from build123d import *

# Parameters (mm, degrees)
F0_W         = 61.9125
F0_H         = 25.4
F1_DEPTH     = 73.025
F3_T         = -2.54
F4_W         = 56.8325
F4_H         = 67.945
F5_DEPTH     = 2.54
F6_T1_DEPTH  = 50.8
F6_T3_DEPTH  = 87.3125
F6_T8_DEPTH  = 87.3125
F6_T14_DEPTH = 87.3125
F6_T20_DEPTH = 87.3125
F6_T27_DEPTH = 87.3125
F6_T33_DEPTH = 87.3125
F7_T1_DEPTH  = 50.8
F7_T3_DEPTH  = 87.3125
F7_T8_DEPTH  = 87.3125
F7_T14_DEPTH = 87.3125
F7_T20_DEPTH = 87.3125
F7_T27_DEPTH = 87.3125
F7_T33_DEPTH = 87.3125
F2_R         = 4.7625
F8_DEPTH     = 61.9135
F10_DEPTH    = 19.05


# Not quite as in the source:
# - a fillet or chamfer that OpenCascade refuses, or shapes differently, is made with other operations: its cross-section is extruded or revolved along the edge and cut away or added


with BuildPart() as f1:
    # F0 (on Front) → F1 (new body)
    with BuildSketch(Plane.XZ):
        Rectangle(F0_W, F0_H)
    extrude(amount=F1_DEPTH)

    # F3
    f3_openings = [f1.faces().sort_by_distance(p)[0] for p in [
        (0, -36.5125, -12.7),
    ]]
    offset(amount=F3_T, openings=f3_openings)

    # F4 (on face) → F5 (join)
    with BuildSketch(Plane.XY.offset(12.7)):
        with Locations((0, -36.5125)):
            Rectangle(F4_W, F4_H)
    extrude(amount=F5_DEPTH)

    # F6: fillet of radius 5.08 on 4 edges, made by hand

    # F6_s2 → F6_t1 (cut)
    with BuildSketch(Plane.XY.offset(-25.4)):
        with BuildLine():
            ThreePointArc((-25.87625, 0), (-29.4683524484, -1.4878975516), (-30.95625, -5.08))
            Line((-30.95625, -5.08), (-30.95625, 0))
            Line((-30.95625, 0), (-25.87625, 0))
        make_face()
        with BuildLine():
            ThreePointArc((30.95625, -5.08), (29.4683524484, -1.4878975516), (25.87625, 0))
            Line((25.87625, 0), (30.95625, 0))
            Line((30.95625, 0), (30.95625, -5.08))
        make_face()
    extrude(amount=F6_T1_DEPTH, mode=Mode.SUBTRACT)

    # F6_s4 → F6_t3 (cut)
    with BuildSketch(Plane.YZ.offset(-43.65625)):
        with BuildLine():
            ThreePointArc((0, -7.62), (-1.4878975516, -11.2121024484), (-5.08, -12.7))
            Line((-5.08, -12.7), (0, -12.7))
            Line((0, -12.7), (0, -7.62))
        make_face()
    extrude(amount=F6_T3_DEPTH, mode=Mode.SUBTRACT)


with BuildPart() as f6_tool6:
    # F6_s7 → F6_t8 (new body)
    with BuildSketch(Plane.YZ.offset(43.65625)):
        with BuildLine():
            ThreePointArc((-5.08, 12.7), (-1.4878975516, 11.2121024484), (0, 7.62))
            Line((0, 7.62), (0, 12.7))
            Line((0, 12.7), (-5.08, 12.7))
        make_face()
    extrude(amount=-F6_T8_DEPTH)

    split(bisect_by=Plane.XZ.offset(2.54), keep=Keep.TOP)

    split(bisect_by=Plane.YZ.offset(28.41625), keep=Keep.TOP)


with BuildPart() as f1_1:
    add(f1.part)

    # F6_t5: cut F6_tool6
    add(f6_tool6.part, mode=Mode.SUBTRACT)


with BuildPart() as f6_tool12:
    # F6_s13 → F6_t14 (new body)
    with BuildSketch(Plane.YZ.offset(43.65625)):
        with BuildLine():
            ThreePointArc((-5.08, 12.7), (-1.4878975516, 11.2121024484), (0, 7.62))
            Line((0, 7.62), (0, 12.7))
            Line((0, 12.7), (-5.08, 12.7))
        make_face()
    extrude(amount=-F6_T14_DEPTH)

    split(bisect_by=Plane.XZ.offset(2.54), keep=Keep.BOTTOM)

    split(bisect_by=Plane.YZ.offset(28.41625), keep=Keep.TOP)


with BuildPart() as f1_2:
    add(f1_1.part)

    # F6_t11: cut F6_tool12
    add(f6_tool12.part, mode=Mode.SUBTRACT)


with BuildPart() as f6_tool18:
    # F6_s19 → F6_t20 (new body)
    with BuildSketch(Plane.YZ.offset(43.65625)):
        with BuildLine():
            ThreePointArc((-5.08, 12.7), (-1.4878975516, 11.2121024484), (0, 7.62))
            Line((0, 7.62), (0, 12.7))
            Line((0, 12.7), (-5.08, 12.7))
        make_face()
    extrude(amount=-F6_T20_DEPTH)

    split(bisect_by=Plane.YZ.offset(-28.41625), keep=Keep.TOP)

    split(bisect_by=Plane.XZ.offset(2.54), keep=Keep.BOTTOM)

    split(bisect_by=Plane.YZ.offset(28.41625), keep=Keep.BOTTOM)


with BuildPart() as f1_3:
    add(f1_2.part)

    # F6_t17: cut F6_tool18
    add(f6_tool18.part, mode=Mode.SUBTRACT)


with BuildPart() as f6_tool25:
    # F6_s26 → F6_t27 (new body)
    with BuildSketch(Plane.YZ.offset(43.65625)):
        with BuildLine():
            ThreePointArc((-5.08, 12.7), (-1.4878975516, 11.2121024484), (0, 7.62))
            Line((0, 7.62), (0, 12.7))
            Line((0, 12.7), (-5.08, 12.7))
        make_face()
    extrude(amount=-F6_T27_DEPTH)

    split(bisect_by=Plane.YZ.offset(-28.41625), keep=Keep.BOTTOM)

    split(bisect_by=Plane.XZ.offset(2.54), keep=Keep.TOP)


with BuildPart() as f1_4:
    add(f1_3.part)

    # F6_t24: cut F6_tool25
    add(f6_tool25.part, mode=Mode.SUBTRACT)


with BuildPart() as f6_tool31:
    # F6_s32 → F6_t33 (new body)
    with BuildSketch(Plane.YZ.offset(43.65625)):
        with BuildLine():
            ThreePointArc((-5.08, 12.7), (-1.4878975516, 11.2121024484), (0, 7.62))
            Line((0, 7.62), (0, 12.7))
            Line((0, 12.7), (-5.08, 12.7))
        make_face()
    extrude(amount=-F6_T33_DEPTH)

    split(bisect_by=Plane.YZ.offset(-28.41625), keep=Keep.BOTTOM)

    split(bisect_by=Plane.XZ.offset(2.54), keep=Keep.BOTTOM)


with BuildPart() as f1_5:
    add(f1_4.part)

    # F6_t30: cut F6_tool31
    add(f6_tool31.part, mode=Mode.SUBTRACT)

    # F7: fillet of radius 5.08 on 4 edges, made by hand

    # F7_s2 → F7_t1 (cut)
    with BuildSketch(Plane.XY.offset(-25.4)):
        with BuildLine():
            ThreePointArc((-25.87625, -73.025), (-29.4683524484, -71.5371024484), (-30.95625, -67.945))
            Line((-30.95625, -67.945), (-30.95625, -73.025))
            Line((-30.95625, -73.025), (-25.87625, -73.025))
        make_face()
        with BuildLine():
            ThreePointArc((30.95625, -67.945), (29.4683524484, -71.5371024484), (25.87625, -73.025))
            Line((25.87625, -73.025), (30.95625, -73.025))
            Line((30.95625, -73.025), (30.95625, -67.945))
        make_face()
    extrude(amount=F7_T1_DEPTH, mode=Mode.SUBTRACT)

    # F7_s4 → F7_t3 (cut)
    with BuildSketch(Plane.YZ.offset(-43.65625)):
        with BuildLine():
            ThreePointArc((-67.945, -12.7), (-71.5371024484, -11.2121024484), (-73.025, -7.62))
            Line((-73.025, -7.62), (-73.025, -12.7))
            Line((-73.025, -12.7), (-67.945, -12.7))
        make_face()
    extrude(amount=F7_T3_DEPTH, mode=Mode.SUBTRACT)


with BuildPart() as f7_tool6:
    # F7_s7 → F7_t8 (new body)
    with BuildSketch(Plane.YZ.offset(43.65625)):
        with BuildLine():
            ThreePointArc((-67.945, 12.7), (-71.5371024484, 11.2121024484), (-73.025, 7.62))
            Line((-73.025, 7.62), (-73.025, 12.7))
            Line((-73.025, 12.7), (-67.945, 12.7))
        make_face()
    extrude(amount=-F7_T8_DEPTH)

    split(bisect_by=Plane.YZ.offset(28.41625), keep=Keep.TOP)

    split(bisect_by=Plane.XZ.offset(70.485), keep=Keep.BOTTOM)


with BuildPart() as f1_6:
    add(f1_5.part)

    # F7_t5: cut F7_tool6
    add(f7_tool6.part, mode=Mode.SUBTRACT)


with BuildPart() as f7_tool12:
    # F7_s13 → F7_t14 (new body)
    with BuildSketch(Plane.YZ.offset(43.65625)):
        with BuildLine():
            ThreePointArc((-67.945, 12.7), (-71.5371024484, 11.2121024484), (-73.025, 7.62))
            Line((-73.025, 7.62), (-73.025, 12.7))
            Line((-73.025, 12.7), (-67.945, 12.7))
        make_face()
    extrude(amount=-F7_T14_DEPTH)

    split(bisect_by=Plane.YZ.offset(28.41625), keep=Keep.TOP)

    split(bisect_by=Plane.XZ.offset(70.485), keep=Keep.TOP)


with BuildPart() as f1_7:
    add(f1_6.part)

    # F7_t11: cut F7_tool12
    add(f7_tool12.part, mode=Mode.SUBTRACT)


with BuildPart() as f7_tool18:
    # F7_s19 → F7_t20 (new body)
    with BuildSketch(Plane.YZ.offset(43.65625)):
        with BuildLine():
            ThreePointArc((-67.945, 12.7), (-71.5371024484, 11.2121024484), (-73.025, 7.62))
            Line((-73.025, 7.62), (-73.025, 12.7))
            Line((-73.025, 12.7), (-67.945, 12.7))
        make_face()
    extrude(amount=-F7_T20_DEPTH)

    split(bisect_by=Plane.YZ.offset(28.41625), keep=Keep.BOTTOM)

    split(bisect_by=Plane.XZ.offset(70.485), keep=Keep.TOP)

    split(bisect_by=Plane.YZ.offset(-28.41625), keep=Keep.TOP)


with BuildPart() as f1_8:
    add(f1_7.part)

    # F7_t17: cut F7_tool18
    add(f7_tool18.part, mode=Mode.SUBTRACT)


with BuildPart() as f7_tool25:
    # F7_s26 → F7_t27 (new body)
    with BuildSketch(Plane.YZ.offset(43.65625)):
        with BuildLine():
            ThreePointArc((-67.945, 12.7), (-71.5371024484, 11.2121024484), (-73.025, 7.62))
            Line((-73.025, 7.62), (-73.025, 12.7))
            Line((-73.025, 12.7), (-67.945, 12.7))
        make_face()
    extrude(amount=-F7_T27_DEPTH)

    split(bisect_by=Plane.XZ.offset(70.485), keep=Keep.BOTTOM)

    split(bisect_by=Plane.YZ.offset(-28.41625), keep=Keep.BOTTOM)


with BuildPart() as f1_9:
    add(f1_8.part)

    # F7_t24: cut F7_tool25
    add(f7_tool25.part, mode=Mode.SUBTRACT)


with BuildPart() as f7_tool31:
    # F7_s32 → F7_t33 (new body)
    with BuildSketch(Plane.YZ.offset(43.65625)):
        with BuildLine():
            ThreePointArc((-67.945, 12.7), (-71.5371024484, 11.2121024484), (-73.025, 7.62))
            Line((-73.025, 7.62), (-73.025, 12.7))
            Line((-73.025, 12.7), (-67.945, 12.7))
        make_face()
    extrude(amount=-F7_T33_DEPTH)

    split(bisect_by=Plane.XZ.offset(70.485), keep=Keep.TOP)

    split(bisect_by=Plane.YZ.offset(-28.41625), keep=Keep.BOTTOM)


with BuildPart() as f1_10:
    add(f1_9.part)

    # F7_t30: cut F7_tool31
    add(f7_tool31.part, mode=Mode.SUBTRACT)

    # F2 (on face) → F8 (cut, through all)
    with BuildSketch(Plane.YZ.offset(30.95625)):
        with Locations((-36.5125, 0)):
            Circle(F2_R)
    extrude(amount=-F8_DEPTH, mode=Mode.SUBTRACT)

    # F9 (on face) → F10 (join)
    with BuildSketch(Plane(origin=(0, 0, 10.16), x_dir=(1, 0, 0), z_dir=(0, 0, -1))):
        Polygon((-3.175, 61.9125), (3.175, 61.9125), (3.175, 59.2770799994), (6.35, 59.3725), (6.35, 61.9125), (6.35, 70.485), (0, 70.485), (-6.35, 70.485), (-6.35, 61.9125), (-6.35, 59.3725), (-3.175, 59.3725), align=None)
        Polygon((3.175, 13.6525), (3.175, 11.1125), (-3.175, 11.1125), (-3.175, 13.6525), (-6.35, 13.6525), (-6.35, 11.1125), (-6.35, 2.54), (6.35, 2.54), (6.35, 11.1125), (6.35, 13.6525), align=None)
    extrude(amount=F10_DEPTH)


solid = f1_10.part
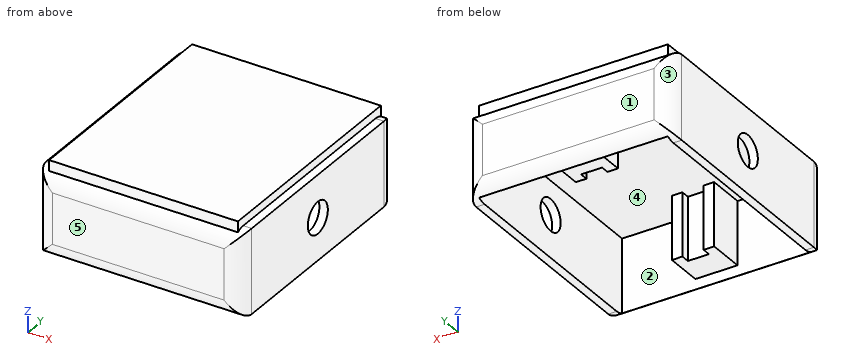
Read the model definition and answer for the solid it produces. Units are mm, in the model's axes. Face numbers are marked on the shaded views. A direction names the side the tool comes from. Give positions to 0.01 mm unless a question says otherwise; leave off trailing zeros. Write each loop counter-clockwise with the first axis right and the second up, starting at its lowest first coordinate (ties: lowest second). Pieces come first, ordered by that corner, then holes. Notation, with made-up numbers: (53, 66.25) -> (57, 66.25) arc R31 cw to (57, 100.25) -> close; hole circle Ø3 at (-16.5, 6.25). An arc over 180 degrees is marked (long way). Answer as a JSON object with one key per item and string values. Group by question number.
1) The mould has two halves that part along Y. Classify the marked faces 3, 4 and 5: +Y half, -Y half, draft (parallel to the pull), parting line (faces both ways), or undercut.
2) A tool of negligible diameter and unlimited length cuts with its end or side. For the marked faces 1 and 2, from which of +Z, -Z, +X, -X, +Y, -Y can it reach the whole face along a straight path? Write none if from no direction.
3) Find section B-B (x = -1). Write down the section's boundary in (y, z) (1 decimal).
4) Find section C-C (z = -10.5). Write down the section's boundary in (x, y) (3 decimals), and give its area (3 significant figures).
5) Each of these flat-tipped pins is pushed along its axis until it touches: P1, Ø5.5, axis at x = 0.5, y = -65, coming from the -Z side; P2, Ø6, axis at x = 3, y = -37.5, coming from the -Z side; P3, Ø1, axis at y = -31, z = 14, coming from the +X side. Where does it stop, or does it pass through?
6) Find section A-A (y = -56.5). Write down the section's boundary in (x, z), and give its area (3 significant figures).
7) Consider L1, parallel to X at y = -10, z = 9.25; L2, parallel to X at y = -30, z = -0.5; L3, parallel to Y at x = 17, z = 7.5 (3 decimals). Determine where each line is inside the solid, lowest interval first. Write a range as from..to.
8) Find section D-D (x = 17). Write down the section's boundary in (y, z) (3 decimals).
Values follow:
{
 "1": {"face 3": "+Y half", "face 4": "undercut", "face 5": "-Y half"},
 "2": {"face 1": "+Z, -Z, +X, -X, +Y", "face 2": "-Z"},
 "3": {"outline": "(-73, -7.6) arc R5.1 ccw to (-70.5, -12) -> (-70.5, -8.9) -> (-61.9, -8.9) -> (-61.9, 10.2) -> (-11.1, 10.2) -> (-11.1, -8.9) -> (-2.5, -8.9) -> (-2.5, -12) arc R5.1 ccw to (0, -7.6) -> (0, 7.6) arc R5.1 ccw to (-2.5, 12) -> (-2.5, 15.2) -> (-70.5, 15.2) -> (-70.5, 12) arc R5.1 ccw to (-73, 7.6) -> close"},
 "4": {"outline": "(-30.956, -67.945) arc R5.08 ccw to (-28.756, -72.13) -> (28.756, -72.13) arc R5.08 ccw to (30.956, -67.945) -> (30.956, -5.08) arc R5.08 ccw to (28.756, -0.895) -> (-28.756, -0.895) arc R5.08 ccw to (-30.956, -5.08) -> close; hole (-28.416, -70.485) -> (28.416, -70.485) -> (28.416, -2.54) -> (-28.416, -2.54) -> close", "area": "538 mm2"},
 "5": {"P1": "stops at z = -8.89", "P2": "stops at z = 10.16", "P3": "stops at x = 28.42"},
 "6": {"outline": "(-30.96, -12.7) -> (-28.42, -12.7) -> (-28.42, 10.16) -> (28.42, 10.16) -> (28.42, -12.7) -> (30.96, -12.7) -> (30.96, 12.7) -> (28.42, 12.7) -> (28.42, 15.24) -> (-28.42, 15.24) -> (-28.42, 12.7) -> (-30.96, 12.7) -> close", "area": "418 mm2"},
 "7": {"L1": "x = -30.96..-28.42, -6.35..6.35, 28.42..30.96", "L2": "x = -30.96..-28.42, 28.42..30.96", "L3": "y = -73.025..-70.485, -2.54..0"},
 "8": {"outline": "(-73.025, -7.62) arc R5.08 ccw to (-70.485, -12.019) -> (-70.485, 10.16) -> (-2.54, 10.16) -> (-2.54, -12.019) arc R5.08 ccw to (0, -7.62) -> (0, 7.62) arc R5.08 ccw to (-2.54, 12.019) -> (-2.54, 15.24) -> (-70.485, 15.24) -> (-70.485, 12.019) arc R5.08 ccw to (-73.025, 7.62) -> close"}
}
